Autodesk Inventor part; units mm, degrees
ref_plane "YZ Plane" through (0, 0, 0) normal (1, 0, 0) x (0, 1, 0)
ref_plane "XZ Plane" through (0, 0, 0) normal (0, 1, 0) x (-1, 0, 0)
ref_plane "XY Plane" through (0, 0, 0) normal (0, 0, 1) x (1, 0, 0)
sketch "Sketch1" plane through (0, 0, 0) normal (1, 0, 0) x (0, 1, 0)
  circle A0 centre (0, 0) radius 1.27
  dimension "d0" = 2.54
extrude "Extrusion1" add sketch "Sketch1" along normal blind 25.4
sketch "Sketch2" plane through (25.4, 0, 0) normal (1, 0, 0) x (0, 0, -1)
  circle A0 centre (0, 0) radius 0.7937
  dimension "d3" = 1.5875
extrude "Extrusion2" add sketch "Sketch2" along normal blind 2.2225
sketch "Sketch3" plane through (0, 0, 0) normal (-1, 0, 0) x (0, 0, 1)
  circle A0 centre (0, 0) radius 0.7937
  dimension "d6" = 1.5875
extrude "Extrusion3" add sketch "Sketch3" along normal blind 2.2225
fillet "Fillet1" radius 0.7937 1 edges at (27.6225, 0, 0.7937)
properties part number "Cable (Red)" material "Aluminum 6061"
Build history of the part. All positions in model axes, mm. A direction names the side the tool comes from. Round coordinates to 2 decimals unless told otherwise and drop trailing zeros. Loops run counter-clockwise (first coordinate to the right, second up) from the corner with the lowest first, then second, coordinate; pieces in that order, holes last. Notation, with made-up numbers: (-18, 37) -> (24, 37) arc R23 ccw to (24, 69) -> close; hole circle Ø1 at (9.25, 3.25). An arc over 180 degrees is marked (long way). One line per item, written item: value. Start each with the question number.
Q1. Cut at A-A on z = 0. List the corners of the cut face in (x, y).
Q2. Probe line 1 along X through (y, z) = (0.25, 1); line 2 along Y through (x, z) = (16, 0.1). List the from-to ranges inside material, lowest first.
Q3. Cut at C-C on x = 16.75. List the corners of the cut face in (y, z).
Q4. Drop flat-ended pins along their axis: pin 1 Ø1.5 at (x, z) = (15, -1) entering from +Y; pin 2 Ø1.5 at (y, z) = (-1, 0) entering from +X. Give the stop position or say it passes through.
Q5. 3-axis set-ups, long thin cutter, end or side, ignore diameter. For faces 1 (the face through (26.104, 0.775, 0.172)), 2 (the face through (-1.096, 0.775, -0.172)), 3 (the face through (12.52, -0.17, -1.26)): which of +Z, -Z, +X, -X, +Y, -Y reach the whole face in a straight line?
Computed:
1. outline: (-2.22, -0.79) -> (0, -0.79) -> (0, -1.27) -> (25.4, -1.27) -> (25.4, -0.79) -> (26.83, -0.79) arc R0.79 ccw to (26.83, 0.79) -> (25.4, 0.79) -> (25.4, 1.27) -> (0, 1.27) -> (0, 0.79) -> (-2.22, 0.79) -> close
2. line 1: 0 to 25.4
2. line 2: -1.27 to 1.27
3. outline: circle Ø2.54 at (0, 0)
4. pin 1: y = 1.25
4. pin 2: x = 27.58
5. face 1: +X
5. face 2: -X
5. face 3: +X, -X
